Read the model definition and answer for the solid it produces. Units are mm, in the model's axes. Coordinates: 2 decimals unless noted, no trailing zeros. Write each loop counter-clockwise with the first axis right and the second up, starting at its lowest first coordinate (ties: lowest second). Pieces come first, ordered by that corner, then holes.
1) Find the intervals of material crossed by line 1 (X direction, y = 0.5, z = 4.5); line 2 (X direction, y = 2, z = 3.5); line 3 (Y direction, x = 52, z = 4.25), in increasing order.
2) The part is cut by section B-B (y = 8). Give the number of separate pieces and of enclosed holes in the cut face, then the cut area to 3 significant figures.
3) The part is cut by section D-D (x = -9). Determine the outline of the cut face in (y, z), then the cut area to 3 significant figures.
4) Each of these flat-tipped pins is pushed along its axis until it touches: pin 1 Ø1.9 at (x, z) = (11, 4.5) entering from +Y; pin 2 Ø3 at (y, z) = (1, 2) entering from -X. Where does it stop, or does it pass through?
5) The part is cut by section A-A (y = 0). Determine the outline of the cut face in (x, z) (3 decimals).
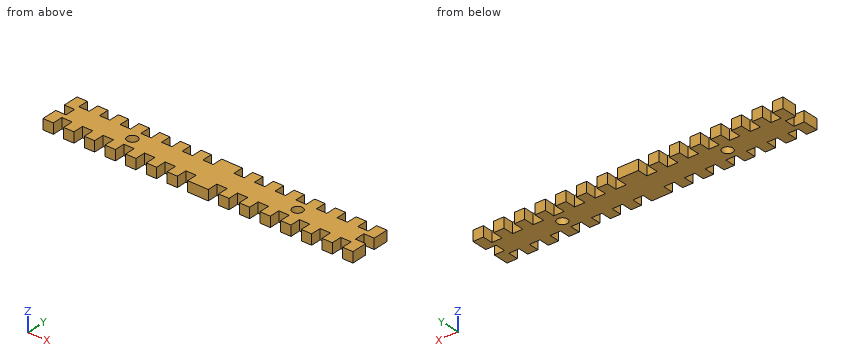
from build123d import *

# Parameters (mm, degrees)
SKETCH1_R           = 3.175
BOSS_EXTRUDE1_DEPTH = 6.35


with BuildPart() as part:
    # Sketch1 → Boss-Extrude1 (new body)
    with BuildSketch(Plane.XY):
        Polygon((-88.9, 12.7), (-95.25, 12.7), (-95.25, 3.175), (-88.9, 3.175), (-88.9, -3.175), (-95.25, -3.175), (-95.25, -12.7), (-88.9, -12.7), (-88.9, -6.35), (-82.55, -6.35), (-82.55, -12.7), (-76.2, -12.7), (-76.2, -6.35), (-69.85, -6.35), (-69.85, -12.7), (-63.5, -12.7), (-63.5, -6.35), (-57.15, -6.35), (-57.15, -12.7), (-50.8, -12.7), (-50.8, -6.35), (-44.45, -6.35), (-44.45, -12.7), (-38.1, -12.7), (-38.1, -6.35), (-31.75, -6.35), (-31.75, -12.7), (-25.4, -12.7), (-25.4, -6.35), (-19.05, -6.35), (-19.05, -12.7), (-12.7, -12.7), (-12.7, -6.35), (-6.35, -6.35), (-6.35, -12.7), (6.35, -12.7), (6.35, -6.35), (12.7, -6.35), (12.7, -12.7), (19.05, -12.7), (19.05, -6.35), (25.4, -6.35), (25.4, -12.7), (31.75, -12.7), (31.75, -6.35), (38.1, -6.35), (38.1, -12.7), (44.45, -12.7), (44.45, -6.35), (50.8, -6.35), (50.8, -12.7), (57.15, -12.7), (57.15, -6.35), (63.5, -6.35), (63.5, -12.7), (69.85, -12.7), (69.85, -6.35), (76.2, -6.35), (76.2, -12.7), (82.55, -12.7), (82.55, -6.35), (88.9, -6.35), (88.9, -12.7), (95.25, -12.7), (95.25, -3.175), (88.9, -3.175), (88.9, 3.175), (95.25, 3.175), (95.25, 12.7), (88.9, 12.7), (88.9, 6.35), (82.55, 6.35), (82.55, 12.7), (76.2, 12.7), (76.2, 6.35), (69.85, 6.35), (69.85, 12.7), (63.5, 12.7), (63.5, 6.35), (57.15, 6.35), (57.15, 12.7), (50.8, 12.7), (50.8, 6.35), (44.45, 6.35), (44.45, 12.7), (38.1, 12.7), (38.1, 6.35), (31.75, 6.35), (31.75, 12.7), (25.4, 12.7), (25.4, 6.35), (19.05, 6.35), (19.05, 12.7), (12.7, 12.7), (12.7, 6.35), (6.35, 6.35), (6.35, 12.7), (-6.35, 12.7), (-6.35, 6.35), (-12.7, 6.35), (-12.7, 12.7), (-19.05, 12.7), (-19.05, 6.35), (-25.4, 6.35), (-25.4, 12.7), (-31.75, 12.7), (-31.75, 6.35), (-38.1, 6.35), (-38.1, 12.7), (-44.45, 12.7), (-44.45, 6.35), (-50.8, 6.35), (-50.8, 12.7), (-57.15, 12.7), (-57.15, 6.35), (-63.5, 6.35), (-63.5, 12.7), (-69.85, 12.7), (-69.85, 6.35), (-76.2, 6.35), (-76.2, 12.7), (-82.55, 12.7), (-82.55, 6.35), (-88.9, 6.35), align=None)
        with Locations((-50.8, 0)):
            Circle(SKETCH1_R, mode=Mode.SUBTRACT)
        with Locations((50.8, 0)):
            Circle(SKETCH1_R, mode=Mode.SUBTRACT)
    extrude(amount=BOSS_EXTRUDE1_DEPTH)


solid = part.part
Reported:
1. line 1: x = -88.9 to -53.94, -47.66 to 47.66, 53.94 to 88.9
1. line 2: x = -88.9 to -53.27, -48.33 to 48.33, 53.27 to 88.9
1. line 3: y = -12.7 to -2.94, 2.94 to 12.7
2. separate pieces: 15
2. enclosed holes: 0
2. area: 645 mm2
3. outline: (-6.35, 0) - (6.35, 0) - (6.35, 6.35) - (-6.35, 6.35) - close
3. area: 80.6 mm2
4. pin 1: stops at y = 6.35
4. pin 2: stops at x = -88.9
5. outline: (-88.9, 0) - (-53.975, 0) - (-53.975, 6.35) - (-88.9, 6.35) - close; (-47.625, 0) - (47.625, 0) - (47.625, 6.35) - (-47.625, 6.35) - close; (53.975, 0) - (88.9, 0) - (88.9, 6.35) - (53.975, 6.35) - close
